Geometry: see drawing. Coordinates: mm, zero at the bounding-box minimum. Give positions to 0.01 mm unless a question says otherwise; leave off trailing zeros. Loops run counter-clockwise (first coordinate to the right, second up) from the corner with the lowest first, then second, coordinate; pieces in that order, holes last. Notation, with made-up numbers: (79, 34.25) -> (129, 34.25) arc R21 ccw to (129, 38.25) -> close; hole circle Ø8 at (-34, 71). An arc over 180 degrees is marked (long way). One line per question, with ' | ' between items.
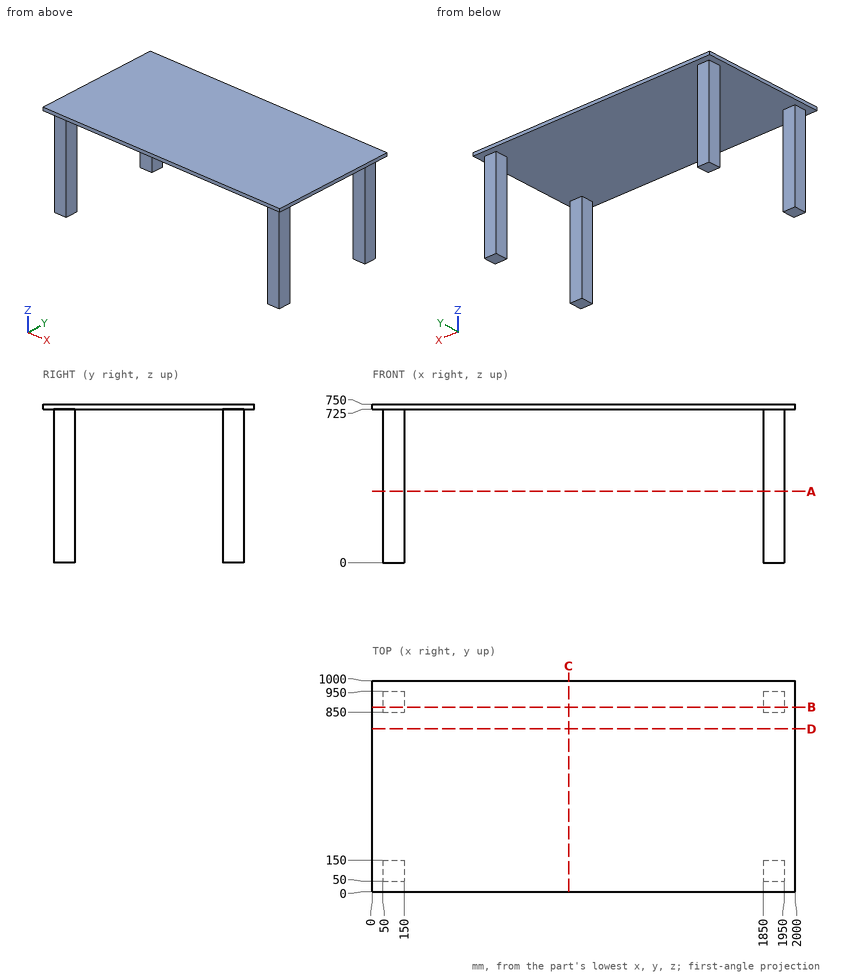
1. Section query C-C (x = 929). Output: boundary loops of the cut face in (y, z), then the cut area to 3 significant figures.
Determined:
outline: (0, 725) -> (1000, 725) -> (1000, 750) -> (0, 750) -> close | area: 25,000 mm2
2. Section query A-A (z = 336.5). Output: boundary loops of the cut face in (x, y).
Determined:
outline: (50, 50) -> (150, 50) -> (150, 150) -> (50, 150) -> close; (50, 850) -> (150, 850) -> (150, 950) -> (50, 950) -> close; (1850, 50) -> (1950, 50) -> (1950, 150) -> (1850, 150) -> close; (1850, 850) -> (1950, 850) -> (1950, 950) -> (1850, 950) -> close
3. Section query B-B (y = 874). Output: boundary loops of the cut face in (x, z), then the cut area to 3 significant figures.
Determined:
outline: (0, 725) -> (50, 725) -> (50, 0) -> (150, 0) -> (150, 725) -> (1850, 725) -> (1850, 0) -> (1950, 0) -> (1950, 725) -> (2000, 725) -> (2000, 750) -> (0, 750) -> close | area: 195,000 mm2
4. Pin query (flat end, axial travel): P1, Ø4, axis at x = 455, y = 814.5, coming from the -Z side. Return the tip coordinate at first contact, or that it passes through.
Determined:
P1: stops at z = 725
5. Ray query, line 1 along X through (y, z) = (139, 498); line 2 along Z through (x, y) = (1760, 871). Return the intervals inside material, ascending. Write a range as from..to.
Determined:
line 1: x = 50..150, 1850..1950 | line 2: z = 725..750
6. Section query D-D (y = 771.5). Output: boundary loops of the cut face in (x, z).
Determined:
outline: (0, 725) -> (2000, 725) -> (2000, 750) -> (0, 750) -> close
